```python
from build123d import *

# Parameters (mm, degrees)
F1_DEPTH = 7.62
F2_SIZE  = 3.81
F3_SIZE  = 3.80999


# Not quite as in the source:
# - a fillet or chamfer is up to 0.001 mm smaller than in the source, because OpenCascade refuses the exact size
# - a feature names something its author has since deleted; it is built from what else it names


with BuildPart() as f1:
    # F0 (on Top) → F1 (new body)
    with BuildSketch(Plane.XY):
        with BuildLine():
            Line((-20.2860954264, -4.4913191196), (-0.4820694779, -51.2720903428))
            Line((-0.4820694779, -51.2720903428), (19.2434711163, -4.6767160388))
            ThreePointArc((19.2434711163, -4.6767160388), (15.0404138493, 4.3253448413), (24.7550324356, 6.4059640289))
            Line((24.7550324356, 6.4059640289), (55.8461389062, 46.4629190132))
            Line((55.8461389062, 46.4629190132), (5.4307896441, 40.2233229702))
            ThreePointArc((5.4307896441, 40.2233229702), (-0.645142483, 32.7880593977), (-7.1331060464, 39.8666485513))
            Line((-7.1331060464, 39.8666485513), (-57.4455202297, 46.8881141422))
            Line((-57.4455202297, 46.8881141422), (-26.8341969161, 6.3469389621))
            ThreePointArc((-26.8341969161, 6.3469389621), (-17.7091606963, 4.4627734196), (-20.2860954264, -4.4913191196))
        make_face()
    extrude(amount=F1_DEPTH)

    # F2
    f2_edges = [f1.edges().sort_by_distance(p)[0] for p in [
        (-32.289313, 43.377381, 0),
        (30.638464, 43.343121, 0),
        (-42.139859, 26.617527, 0),
        (40.300586, 26.434442, 0),
        (9.380701, -27.974403, 0),
        (-10.384082, -27.881705, 0),
        (15.040414, 4.325345, 0),
    ]]
    chamfer(f2_edges, length=F2_SIZE)

    # F3 (size 3.81 in the source; OpenCascade refuses exactly that, so slightly less here)
    f3_edges = [f1.edges().sort_by_distance(p)[0] for p in [
        (-32.289313, 43.377381, 7.62),
        (-42.139859, 26.617527, 7.62),
        (-10.384082, -27.881705, 7.62),
        (9.380701, -27.974403, 7.62),
        (40.300586, 26.434442, 7.62),
        (30.638464, 43.343121, 7.62),
        (15.040414, 4.325345, 7.62),
        (-0.645142, 32.788059, 7.62),
        (-17.709161, 4.462773, 7.62),
        (-17.729481, 4.496175, 0),
        (-0.591, 32.789828, 0),
    ]]
    chamfer(f3_edges, length=F3_SIZE)


solid = f1.part
```
Check sheet for the modelled part. Datum: model origin and axes. Units: mm. A direction names the side the tool comes from. Coordinates: 2 decimals unless noted, no trailing zeros. Loops run counter-clockwise (first coordinate to the right, second up) from the corner with the lowest first, then second, coordinate; pieces in that order, holes last.
1) Release check for a two-part mould opening along Y. For faces 3 (the face through (7.464, -27.548, 1.878)), 4 (the face through (-17.23, 4.94, 3.15)), 5 (the face through (-1, 10, 7.62)) record: released by +Y, released by -Y, zero draft, split by the parting line, or undercut.
2) Material ranges on probe 1 along X at (y, z) = (34, 4.5); probe 2 along X at (y, z) = (0, 4.25); probe 3 along X at (y, z) = (-19.5, 1.25), recorded low to high.
3) Sectioned sample at A-A (z = 5.25). Record the boundary of the cut face in (x, y).
4) Gauge pin test, flat ends, axial feed: pin 1 (16.5 mm diameter, centred on x = -0.83, y = 39.14, fed in from +Z); pin 2 (3 mm diameter, centred on x = -25.5, z = 5.5, fed in from +Y); pin 3 (1.5 mm diameter, centred on y = -29.5, z = 1, fed in from -X). Record the tip position at first contact, or that the pin passes through.
5) Access from +Z, -Z, +X, -X, +Y, -Y to the whole of each face (thin tool, end or side, straight path). Record for faces 1 (the face through (-32.197, 41.468, 5.688)), 2 (the face through (-1, 10, 0)).
Check sheet entries:
1. face 3: released by -Y
1. face 4: undercut
1. face 5: zero draft
2. probe 1: x = -46.85 to -5.64, 3.99 to 45.3
2. probe 2: x = -16.46 to 14.1
2. probe 3: x = -11.15 to 10.19
3. outline: (-54.2, 44.98) - (-26.45, 8.23) arc R7.79 cw to (-18.48, -5.06) - (-0.48, -47.58) - (17.33, -5.51) arc R7.79 cw (long way) to (24.44, 8.35) - (52.58, 44.61) - (6.96, 38.96) arc R7.79 cw to (-8.6, 38.62) - close
4. pin 1: stops at z = 5.71
4. pin 2: stops at y = 42.25
4. pin 3: stops at x = -7.52
5. face 1: +Z, +Y
5. face 2: -Z, +X, -X, +Y, -Y
